The listing builds one solid part. Answer for the finished solid, in the listing's coordinates (mm). Round coordinates to 2 decimals unless told otherwise and drop trailing zeros. Write each loop counter-clockwise with the first axis right and the second up, starting at its lowest first coordinate (ties: lowest second). Pieces come first, ordered by that corner, then holes.
Item 1: For a pull along X with two mould halves and no side action, classify faces 1 (the face through (-0.8, -62.6, 6.3)), 2 (the face through (3, -127, -4)), 3 (the face through (-0.69, -25.05, -4.7)) as +X half, -X half, draft (parallel to the pull), parting line (faces both ways), or undercut.
Item 2: Find section B-B on z = 0. Give the vertices of the cut face in (x, y) (3 decimals), then the cut area to 3 significant figures.
Item 3: Find the intervals of material crossed by probe 1 along Z at (x, y) = (0, -73) (3 decimals); probe 2 along Y at (x, z) = (0, -5); probe 3 along X at (y, z) = (-40, -0.25), in increasing order.
Item 4: Find section A-A on x = 0. Give the vertices of the cut face in (y, z) (3 decimals), then the cut area to 3 significant figures.
Item 5: Find section C-C on y = -10. Give the vertices of the cut face in (x, z) (3 decimals).
Item 6: Each of these flat-tipped pins is pushed along its axis until it touches: pin 1 (2 mm diameter, centred on x = 2, y = -48.5, fed in from +Z); pin 2 (2 mm diameter, centred on x = -3.5, y = -95.5, fed in from +Z); pin 3 (5 mm diameter, centred on x = -2, z = 1, fed in from -Y); pin 4 (1.5 mm diameter, centred on x = 2.5, z = -0.5, fed in from +Y). Where does it stop, or does it pass through?
```python
from build123d import *

# Parameters (mm, degrees)
F0_R     = 6.35
F1_DEPTH = 127
F2_R     = 4.445
F3_DEPTH = 127
F4_R     = 3.1877
F5_DEPTH = 6.351


with BuildPart() as f1:
    # F0 (on Front) → F1 (new body)
    with BuildSketch(Plane.XZ):
        Circle(F0_R)
    extrude(amount=F1_DEPTH)

    # F2 (on Front) → F3 (cut)
    with BuildSketch(Plane.XZ):
        Circle(F2_R)
    extrude(amount=F3_DEPTH, mode=Mode.SUBTRACT)

    # F4 (on Top) → F5 (cut, through all)
    with BuildSketch(Plane.XY):
        with Locations((0, -21.939068)):
            Circle(F4_R)
    extrude(amount=-F5_DEPTH, mode=Mode.SUBTRACT)


solid = f1.part
```
Check values:
1. face 1: parting line
1. face 2: draft
1. face 3: undercut
2. outline: (-6.35, -127) - (-4.445, -127) - (-4.445, 0) - (-6.35, 0) - close; (4.445, -127) - (6.35, -127) - (6.35, 0) - (4.445, 0) - close
2. area: 484 mm2
3. probe 1: z = -6.35 to -4.445, 4.445 to 6.35
3. probe 2: y = -127 to -25.13, -18.75 to 0
3. probe 3: x = -6.35 to -4.44, 4.44 to 6.35
4. outline: (-127, -6.35) - (-25.127, -6.35) - (-25.127, -4.445) - (-127, -4.445) - close; (-127, 4.445) - (0, 4.445) - (0, 6.35) - (-127, 6.35) - close; (-18.751, -6.35) - (0, -6.35) - (0, -4.445) - (-18.751, -4.445) - close
4. area: 472 mm2
5. outline: circle Ø12.7 at (0, 0); hole circle Ø8.89 at (0, 0)
6. pin 1: stops at z = 6.27
6. pin 2: stops at z = 5.84
6. pin 3: stops at y = -127
6. pin 4: passes through
